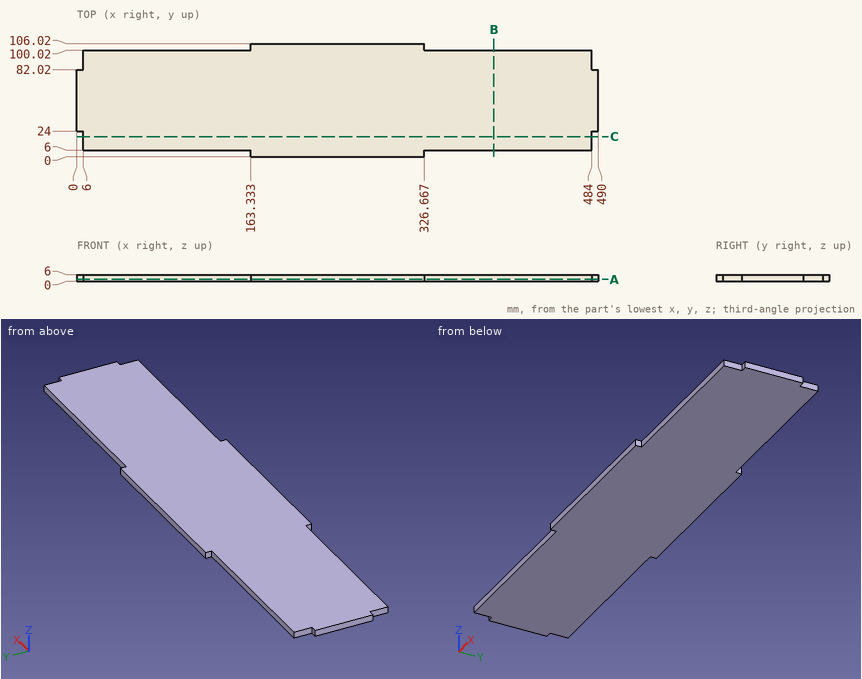
Verification items for this drawing (mm, ordinates from the low corner). Coordinates: 2 decimals unless noted, no trailing zeros. Order: outer loops, then holes, each group sorted by start corner. A loop starts at its lowest first (then second) coordinate and runs counter-clockwise, first axis right, second up. Notation, with made-up numbers: M 58.5,-15 L 66.5,-15 A16 cw 66.5,-6 Z; hole C -6.5,69 d10. An arc over 180 degrees is marked long. One line per item, written item: value. Start each with the question number.
Item 1: Sectioned sample at C-C on y = 19. Record the cut outline in (x, z).
Item 2: Depth check by flat-ended pin: P1, Ø3, axis at x = 487.5, z = 4.5, coming from the +Y side; P2, Ø3, axis at y = 3.5, z = 2, coming from the +X side; P3, Ø3, axis at x = 94.5, z = 3.5, coming from the -Y side. Enter the tip coordinate at first touch or a pass-through.
Item 3: Sectioned sample at B-B on x = 392. Record the cut outline in (y, z), then the cut area to 3 significant figures.
Item 4: Sectioned sample at A-A on z = 1.75. Record the cut outline in (x, y).
Item 5: Thickness scan on probe 1 along X at (y, z) = (11, 3.8); probe 2 along Y at (x, z) = (348.5, 1.25). Record the ranges inside material, lowest first.
Calculated:
1. outline: M 6,0 L 484,0 L 484,6 L 6,6 Z
2. P1: y = 82.02
2. P2: x = 326.67
2. P3: y = 6
3. outline: M 6,0 L 100.02,0 L 100.02,6 L 6,6 Z
3. area: 564 mm^2
4. outline: M 0,24 L 6,24 L 6,6 L 163.33,6 L 163.33,0 L 326.67,0 L 326.67,6 L 484,6 L 484,24 L 490,24 L 490,82.02 L 484,82.02 L 484,100.02 L 326.67,100.02 L 326.67,106.02 L 163.33,106.02 L 163.33,100.02 L 6,100.02 L 6,82.02 L 0,82.02 Z
5. probe 1: 6 to 484
5. probe 2: 6 to 100.02
